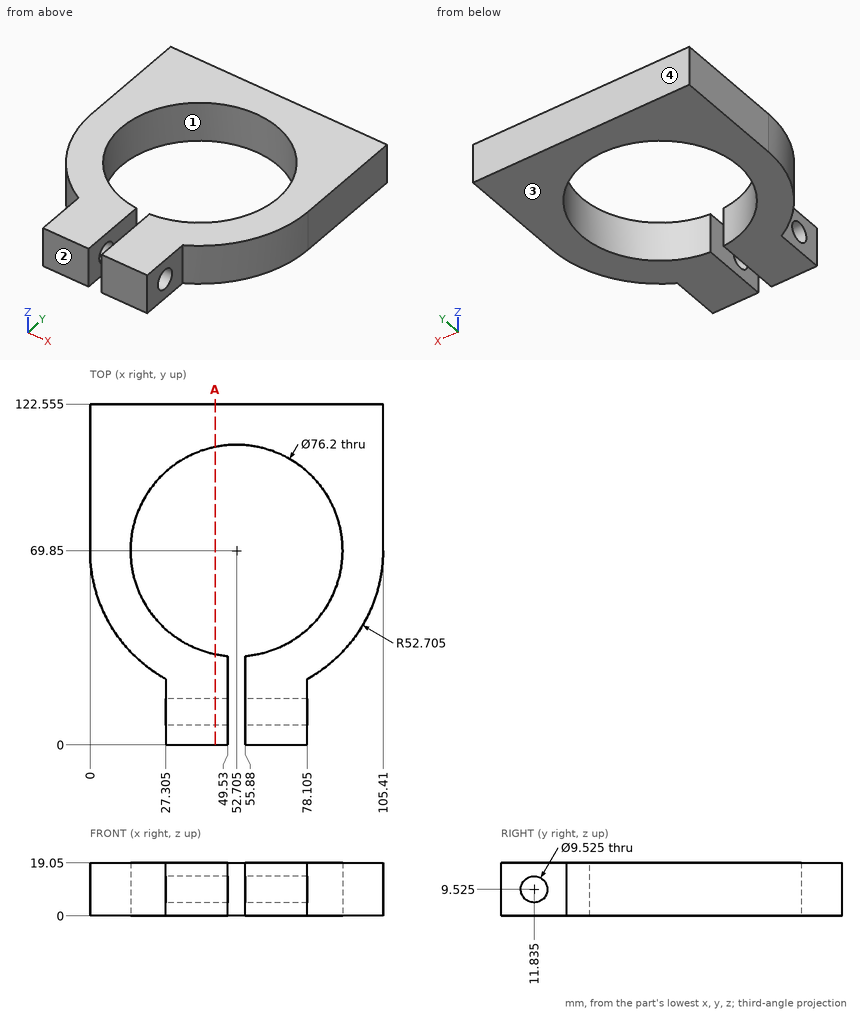
Could you check a few things on this drawing? It's one solid part, dimensions in mm from its lowest x, y, z. Round coordinates to 2 decimals unless told otherwise and drop trailing zeros.
Q1. Will these pins go through, and if not, where does the flat tip stop? P1, Ø2, axis at y = 39, z = 12.5, coming from the -X side; P2, Ø1.5, axis at x = 74, y = 21, coming from the -Z side; P3, Ø9.5, axis at y = 11.5, z = 11.5, coming from the -X side (3 decimals); P4, Ø8, axis at y = 31.5, z = 13.5, coming from the -X side.
Q2. If we mould it in two halves opening along Y, with no side actions, what happens to the marked faces 1, 2, 3 and 4? For each: +Y half, -Y half, draft (parallel to the pull), parting line (faces both ways), or undercut.
Q3. Please list where these lines run through material, in increasing order: probe 1 along X at (y, z) = (20, 2) (1 decimal); probe 2 along Y at (x, z) = (48, 13) (1 decimal); probe 3 along Y at (x, z) = (58, 10.5) (1 decimal).
Q4. If we section it at A-A on x = 45: Give the number of separate pieces and of enclosed holes in the cut face, plus the area to 3 significant figures.
Answer below:
1. P1: stops at x = 9.27
1. P2: stops at z = 0
1. P3: stops at x = 27.305
1. P4: stops at x = 12.73
2. face 1: undercut
2. face 2: -Y half
2. face 3: draft
2. face 4: +Y half
3. probe 1: x = 27.3 to 49.5, 55.9 to 78.1
3. probe 2: y = 0 to 8.6, 15.1 to 32, 107.7 to 122.6
3. probe 3: y = 0 to 7.2, 16.5 to 32.1, 107.6 to 122.6
4. separate pieces: 2
4. enclosed holes: 1
4. area: 842 mm2
